```python
from build123d import *

# Parameters (mm, degrees)
SKETCH1_R           = 1
BOSS_EXTRUDE1_DEPTH = 11
SKETCH2_R           = 1.25
BOSS_EXTRUDE2_DEPTH = 1
CHAMFER1_SIZE       = 0.5
CHAMFER2_SIZE       = 0.5
FILLET1_R           = 0.5


# Some blends are built 0.0001 mm under size
with BuildPart() as part:
    # Sketch1 → Boss-Extrude1 (new body)
    with BuildSketch(Plane(origin=(0, 0, 0), x_dir=(1, 0, 0), z_dir=(0, 1, 0))):
        with Locations(Location((0, 0, 0), (0, 0, 270))):
            Circle(SKETCH1_R)
    extrude(amount=-BOSS_EXTRUDE1_DEPTH)

    # Sketch2 → Boss-Extrude2 (add)
    with BuildSketch(Plane(origin=(0, 0, 0), x_dir=(1, 0, 0), z_dir=(0, 1, 0))):
        with Locations(Location((0, 0, 0), (0, 0, 270))):
            Circle(SKETCH2_R)
    extrude(amount=BOSS_EXTRUDE2_DEPTH)

    # Chamfer1
    # the kernel refuses this chamfer: 0.5 mm, written as the material it takes off along each edge
    with BuildSketch(Plane(origin=(0, 0, 0), x_dir=(0, 0, 1), z_dir=(-1, 0, 0))) as chamfer1_piece_1_section:
        Polygon((1.25, CHAMFER1_SIZE), (1.25 - CHAMFER1_SIZE, 0), (1.25, 0), align=None)
    chamfer1_piece_1 = revolve(axis=Axis((0, 0, 0), (0, 1, 0)), mode=Mode.PRIVATE)
    chamfer1_piece_1 = chamfer1_piece_1 - Plane(origin=(0, 0.375686262, 0), x_dir=(0, 0, 1), z_dir=(0, 1, 0)) * Cylinder(1, 5, mode=Mode.PRIVATE)
    add(chamfer1_piece_1, mode=Mode.SUBTRACT)

    # Chamfer2
    chamfer2_edges = [part.edges().sort_by_distance(p)[0] for p in [
        (0, -11, -1),
    ]]
    chamfer(chamfer2_edges, length=CHAMFER2_SIZE)

    # Fillet1
    fillet1_edges = [part.edges().sort_by_distance(p)[0] for p in [
        (0, 1, -1.25),
    ]]
    fillet(fillet1_edges, radius=FILLET1_R - 0.0001)  # a hair under: the kernel refuses the full size


solid = part.part
```
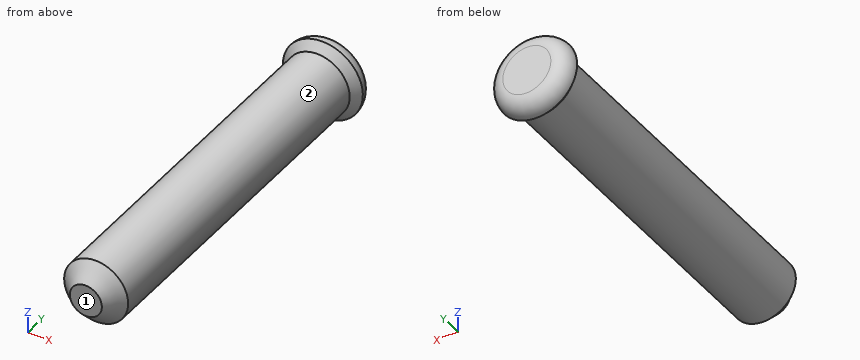
Here's how the part is built. I have some questions about the finished solid (model axes, mm). Face numbers are marked on the shaded views. A direction names the side the tool comes from. Coordinates: 2 decimals unless noted, no trailing zeros. Write each loop counter-clockwise with the first axis right and the second up, starting at its lowest first coordinate (ties: lowest second). Pieces come first, ordered by that corner, then holes. Notation, with made-up numbers: (36, -29.75) - (94, -29.75) arc R16 cw to (94, -12.75) - close; hole circle Ø1 at (-30.5, -11.5). An arc over 180 degrees is marked (long way). One line per item, written item: value.
1) Suppose I cut it at C-C on y = -7.5. Write out the boundary of the cut face in (x, z).
Model answer:
outline: circle Ø2 at (0, 0)
2) I'm going to push flat-ended pins straight in: P1, Ø1, axis at x = -1, z = -0.5, coming from the -Y side; P2, Ø1, axis at x = 0.5, y = -5, coming from the +Z side. Where does each tip first touch, or does it pass through?
Model answer:
P1: stops at y = -10.88
P2: stops at z = 1
3) On a 3-axis mill with a long thin cutter (end or side, diameter ignored), from which of +Z, -Z, +X, -X, +Y, -Y can I reach the whole of each face in a straight line? I mean the marked faces 1 and 2. Say none if no direction works.
Model answer:
face 1: +Z, -Z, +X, -X, -Y
face 2: -Y
4) I need wall thicknesses on line 1 along Z through (x, y) = (0.7, -4.75); line 2 along Y through (x, z) = (-0.35, -0.6); line 3 along Z through (x, y) = (-0.5, -4.75). Which ranges of each line are inside material? Lowest first, please.
Model answer:
line 1: z = -0.71 to 0.71
line 2: y = -10.81 to 1
line 3: z = -0.87 to 0.87
